from build123d import *

# Parameters (mm, degrees)
SKETCH_2_W          = 130
SKETCH_2_H          = 128
EXTRUDE_1_DEPTH     = 3
SKETCH_3_R          = 2.5
CUT_EXTRUDE_1_DEPTH = 92.268833673


with BuildPart() as part:
    # 草圖2 → 填料-伸長1 (new body)
    with BuildSketch(Plane.XY):
        Rectangle(SKETCH_2_W, SKETCH_2_H)
        Polygon((0, 19.647280252), (30.826980994, 50), (-30.826980994, 50), align=None, mode=Mode.SUBTRACT)
        Polygon((-51, 30.568104363), (-19.954269006, 0), (-51, -30.568104363), align=None, mode=Mode.SUBTRACT)
        Polygon((19.954269006, 0), (51, 30.568104363), (51, -30.568104363), align=None, mode=Mode.SUBTRACT)
        Polygon((30.826980994, -50), (0, -19.647280252), (-30.826980994, -50), align=None, mode=Mode.SUBTRACT)
    extrude(amount=EXTRUDE_1_DEPTH)

    # 草圖3 → 除料-伸長1 (cut, through all)
    with BuildSketch(Plane(origin=(0, 0, 0), x_dir=(-1, 0, 0), z_dir=(0, 0, -1))):
        with Locations((-52, -54)):
            Circle(SKETCH_3_R)
        with Locations((-52, -36)):
            Circle(SKETCH_3_R)
        with Locations((52, -54)):
            Circle(SKETCH_3_R)
        with Locations((52, -36)):
            Circle(SKETCH_3_R)
        with Locations((-52, 54)):
            Circle(SKETCH_3_R)
        with Locations((-52, 36)):
            Circle(SKETCH_3_R)
        with Locations((52, 54)):
            Circle(SKETCH_3_R)
        with Locations((52, 36)):
            Circle(SKETCH_3_R)
    extrude(amount=-CUT_EXTRUDE_1_DEPTH, mode=Mode.SUBTRACT)


solid = part.part
Could you check a few things on this model? Use its own coordinates, in mm. A direction names the side the tool comes from. Round coordinates to 2 decimals unless told otherwise and drop trailing zeros. Order: outer loops, then holes, each group sorted by start corner. A loop starts at its lowest first (then second) coordinate and runs counter-clockwise, first axis right, second up. Notation, with made-up numbers: M 5.5,-22 L 60.5,-22 A19 cw 60.5,6 Z; hole C 36,29 d1. An arc over 180 degrees is marked long. One line per item, written item: value.
(1) Imagine slicing it at A-A (y = 54). Write out the boundary of the cut face in (x, z).
Ans:
outline: M -65,0 L -54.5,0 L -54.5,3 L -65,3 Z; M -49.5,0 L 49.5,0 L 49.5,3 L -49.5,3 Z; M 54.5,0 L 65,0 L 65,3 L 54.5,3 Z
(2) Imagine slicing it at D-D (y = -48.5). Write out the boundary of the cut face in (x, z), and give its area (3 significant figures).
Ans:
outline: M -65,0 L -29.3,0 L -29.3,3 L -65,3 Z; M 29.3,0 L 65,0 L 65,3 L 29.3,3 Z
area: 214 mm^2
(3) Imagine slicing it at B-B (z = 1.05). Count the separate pieces of the cut face and the enclosed holes in it, and give its area (3 significant figures).
Ans:
separate pieces: 1
enclosed holes: 12
area: 12,700 mm^2
(4) I need wall thicknesses on line 1 along Y through (x, z) = (52, 0.75); line 2 along Y through (x, z) = (-11.5, 2.15); line 3 along X through (y, z) = (29, 0.55). Which ranges of each line are inside material? Lowest first, please. Write a range as from..to.
Ans:
line 1: y = -64..-56.5, -51.5..-38.5, -33.5..33.5, 38.5..51.5, 56.5..64
line 2: y = -64..-50, -30.97..30.97, 50..64
line 3: x = -65..-51, -49.41..-9.5, 9.5..49.41, 51..65
(5) If we mould it in two halves opening along X, with no side actions, what happens to faces 3 (the flat face through (-1, -64, 1)), 4 (the flat face through (-15.629, 35.036, 1.479)), 5 (the flat face through (-65, -1, 1)), 6 (the cylindrical face through (-54.31, 53.04, 1.48))? For each: released by +X, released by -X, zero draft, split by the parting line, or undercut.
Ans:
face 3: zero draft
face 4: undercut
face 5: released by -X
face 6: undercut
(6) Which directions (+Z, -Z, +X, -X, +Y, -Y) give clear straight access to the entire face, cutting with the end or side of a thin tool? Please do faces 1 (the flat face through (-35.26, -15.07, 1.48)), 2 (the flat face through (-1, 1, 0)).
Ans:
face 1: +Z, -Z
face 2: -Z, +X, -X, +Y, -Y
(7) Imagine slicing it at C-C (x = -48). Write out the boundary of the cut face in (y, z).
Ans:
outline: M -64,0 L -27.61,0 L -27.61,3 L -64,3 Z; M 27.61,0 L 64,0 L 64,3 L 27.61,3 Z
